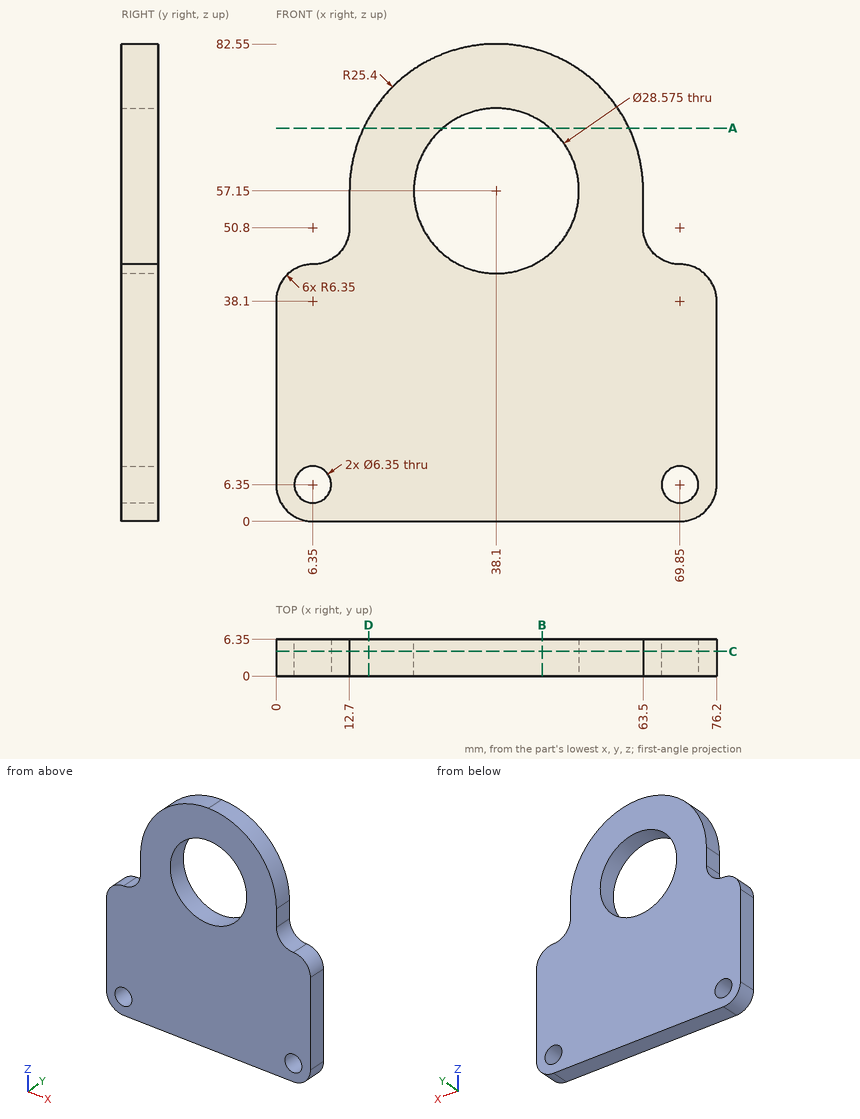
Geometry check sheet. Reference: drawing and pictorial views, mm from the part's lowest x, y, z. Round coordinates to 2 decimals unless told otherwise and drop trailing zeros. Order: outer loops, then holes, each group sorted by start corner. A loop starts at its lowest first (then second) coordinate and runs counter-clockwise, first axis right, second up.
Q1. Depth check by flat-ended pin: P1, Ø1, axis at y = 5.5, z = 47.5, coming from the +X side; P2, Ø4, axis at x = 6.35, z = 6.35, coming from the +Y side; P3, Ø8, axis at x = 23, z = 22, coming from the -Y side; P4, Ø1.9, axis at y = 3.5, z = 55.5, coming from the -X side. Enter the tip coordinate at first touch or a pass-through.
Filled sheet:
P1: stops at x = 64.76
P2: passes through
P3: stops at y = 0
P4: stops at x = 12.7
Q2. Cross-section at A-A, the plane z = 68. Enter the section's corners in (x, y).
Filled sheet:
outline: (15.13, 0) - (28.8, 0) - (28.8, 6.35) - (15.13, 6.35) - close; (47.4, 0) - (61.07, 0) - (61.07, 6.35) - (47.4, 6.35) - close
Q3. Scan lines: L1, parallel to X at y = 5.5, z = 57; L2, parallel to Z at x = 69.5, y = 0.75; L3, parallel to X at y = 4.25, z = 38.5. Record each from-to range of solid material in increasing order.
Filled sheet:
L1: x = 12.7 to 23.81, 52.39 to 63.5
L2: z = 0 to 3.19, 9.51 to 44.46
L3: x = 0.01 to 76.19
Q4. Cross-section at D-D, the plane x = 16. Enter the section's corners in (y, z).
Filled sheet:
outline: (0, 0) - (6.35, 0) - (6.35, 69.67) - (0, 69.67) - close
Q5. Cross-section at B-B, the plane x = 46. Enter the section's corners in (y, z), plus the area to 3 significant figures.
Filled sheet:
outline: (0, 0) - (6.35, 0) - (6.35, 45.25) - (0, 45.25) - close; (0, 69.05) - (6.35, 69.05) - (6.35, 81.29) - (0, 81.29) - close
area: 365 mm2
Q6. Cross-section at C-C, the plane y = 4.25. Give the number of separate pieces and of enclosed holes in the cut face, plus the area to 3 significant figures.
Filled sheet:
separate pieces: 1
enclosed holes: 3
area: 4,320 mm2
